from build123d import *

# Parameters (mm, degrees)
EXTRUDE_1_DEPTH   = 1018.75
FILLET_1_R        = 10
FILLET_2_R        = 8
FILLET_3_R        = 3
FILLET_4_R        = 10
FILLET_5_R        = 3
EXTRUDE_START     = 118.75
EXTRUDE_1_2_DEPTH = 118.75
EXTRUDE_2_DEPTH   = 8


with BuildPart() as part:
    # 草图1 → Extrude 1 (new body)
    with BuildSketch(Plane.XY):
        Polygon((-35, 49.6), (-35, 83.5), (35, 83.5), (35, 49.6), (15, 44.6), (15, -41.6), (67, -54.6), (67, -68.5), (-65, -68.5), (-65, -54.6), (-15, -42.1), (-15, 44.6), align=None)
    extrude(amount=EXTRUDE_1_DEPTH)

    # 圆角1
    fillet_1_edges = [part.edges().sort_by_distance(p)[0] for p in [
        (15, -41.6, 509.375),
        (-15, -42.1, 509.375),
    ]]
    fillet(fillet_1_edges, radius=FILLET_1_R)

    # 圆角2
    fillet_2_edges = [part.edges().sort_by_distance(p)[0] for p in [
        (15, 44.6, 509.375),
        (-15, 44.6, 509.375),
    ]]
    fillet(fillet_2_edges, radius=FILLET_2_R)

    # 圆角3
    fillet_3_edges = [part.edges().sort_by_distance(p)[0] for p in [
        (-35, 49.6, 509.375),
        (35, 49.6, 509.375),
    ]]
    fillet(fillet_3_edges, radius=FILLET_3_R)

    # 圆角4
    fillet_4_edges = [part.edges().sort_by_distance(p)[0] for p in [
        (-35, 83.5, 509.375),
        (35, 83.5, 509.375),
    ]]
    fillet(fillet_4_edges, radius=FILLET_4_R)

    # 圆角5
    fillet_5_edges = [part.edges().sort_by_distance(p)[0] for p in [
        (67, -54.6, 509.375),
        (-65, -54.6, 509.375),
    ]]
    fillet(fillet_5_edges, radius=FILLET_5_R)

    # 草图4 → Extrude 1 2 (add)
    with BuildSketch(Plane.XY.offset(450).offset(EXTRUDE_START)):
        with BuildLine():
            Line((142, -68.5), (142, -58.5))
            ThreePointArc((142, -58.5), (140.535533906, -54.964466094), (137, -53.5))
            Line((137, -53.5), (100.637155323, -53.5))
            ThreePointArc((100.637155323, -53.5), (97.219067588, -52.897695262), (94.212725941, -51.163335247))
            Line((94.212725941, -51.163335247), (69.787274059, -30.686664753))
            ThreePointArc((69.787274059, -30.686664753), (66.780932412, -28.952304738), (63.362844677, -28.35))
            Line((63.362844677, -28.35), (27, -28.35))
            ThreePointArc((27, -28.35), (23.464466094, -29.814466094), (22, -33.35))
            Line((22, -33.35), (22, -43.35))
            Line((22, -43.35), (64.727606875, -54.031901719))
            ThreePointArc((64.727606875, -54.031901719), (66.364616314, -55.096092591), (67, -56.942329219))
            Line((67, -56.942329219), (67, -63.5))
            ThreePointArc((67, -63.5), (68.464466094, -67.035533906), (72, -68.5))
            Line((72, -68.5), (142, -68.5))
        make_face()
    extrude_1_2 = extrude(amount=-EXTRUDE_1_2_DEPTH)

    # 草图5 → 凸台-拉伸2 (add)
    with BuildSketch(Plane(origin=(0, -53.5, 0), x_dir=(1, 0, 0), z_dir=(0, 1, 0))):
        Polygon((124.592080354, -519.375), (130.365583045, -509.375), (124.592080354, -499.375), (113.04507497, -499.375), (107.271572278, -509.375), (113.04507497, -519.375), align=None)
    extrude_2 = extrude(amount=EXTRUDE_2_DEPTH)

    # 镜向1: Extrude 1 2, 凸台-拉伸2 across plane
    add(extrude_1_2.mirror(Plane(origin=(1, 0, 0), x_dir=(0, 0, 1), z_dir=(1, 0, 0))))
    add(extrude_2.mirror(Plane(origin=(1, 0, 0), x_dir=(0, 0, 1), z_dir=(1, 0, 0))))


solid = part.part
Check sheet for the modelled part. Datum: model origin and axes. Units: mm. A direction names the side the tool comes from. Give positions to 0.01 mm unless a question says otherwise; leave off trailing zeros. Loops run counter-clockwise (first coordinate to the right, second up) from the corner with the lowest first, then second, coordinate; pieces in that order, holes last. Notation, with made-up numbers: M 6.5,-4 L 47.5,-4 A17 ccw 47.5,22 Z; hole C -22.5,24 d6. An arc over 180 degrees is marked long. Use a Markdown table: item, result. Add a question column.
Q1. Scan lines: line 1 along X through (y, z) = (28, 599); line 2 along Y through (x, z) = (-83, 535); line 3 along X through (y, z) = (-62, 339.5). Record each from-to range of solid material in increasing order. Write a range as [from, to].
Q2. Sectioned sample at B-B, the plane y = -11. Record the cut outline in (x, z).
Q3. Go/stop test with flat-tipped pins: pin 1 (10 mm diameter, centred on y = 31, z = 828.5, fed in from -X); pin 2 (6.5 mm diameter, centred on x = 121, y = -51, fed in from +Z); pin 3 (9 mm diameter, centred on y = -61, z = 285.5, fed in from -X). Record where each tip stops, or that it passes through.
Q4. Sectioned sample at A-A, the plane z = 108. Record the cut outline in (x, y).
Q5. Tool access check on faces 5 (the flat face through (-43, -28.35, 510)), 6 (the flat face through (-42.932, -49.083, 221.85)), 7 (the flat face through (45, -28.35, 510)), 8 (the flat face through (-117, -45.5, 509)), 9 (the flat face through (119, -45.5, 509)). Record the directions out of +Z, -Z, +X, -X, +Y, -Y that give a thin tool (end or side, any length) a straight path to the whole face; none if there is none.
Q6. Mould release check, pull along Y, two halves, no side actions. Record for faces 1 (the flat face through (-105, -53.5, 510)), 2 (the flat face through (43.4, -48.7, 221.8)), 3 (the flat face through (-42.932, -49.083, 790.6)), 4 (the flat face through (2, 9, 0)): pulls with the +Y half, pulls with the -Y half, needs draft (parallel to the pull), parting line crosses it, or undercut.
Verdict:
| question | item | result |
|---|---|---|
| 1 | line 1 | [-15, 15] |
| 1 | line 2 | [-68.5, -43.44] |
| 1 | line 3 | [-65, 67] |
| 2 | outline | M -15,0 L 15,0 L 15,1018.75 L -15,1018.75 Z |
| 3 | pin 1 | x = -15 |
| 3 | pin 2 | z = 568.75 |
| 3 | pin 3 | x = -65 |
| 4 | outline | M -65,-68.5 L 67,-68.5 L 67,-56.94 A3 ccw 64.73,-54.03 L 22.57,-43.49 A10 cw 15,-33.79 L 15,38.35 A8 cw 21.06,46.11 L 32.73,49.03 A3 ccw 35,51.94 L 35,73.5 A10 ccw 25,83.5 L -25,83.5 A10 ccw -35,73.5 L -35,51.94 A3 ccw -32.73,49.03 L -21.06,46.11 A8 cw -15,38.35 L -15,-34.29 A10 cw -22.57,-43.99 L -62.73,-54.03 A3 ccw -65,-56.94 Z |
| 5 | face 5 | +Z, -Z, -X |
| 5 | face 6 | -Z, -X |
| 5 | face 7 | +Z, -Z, +X |
| 5 | face 8 | +Z, -Z, -X, +Y |
| 5 | face 9 | +Z, -Z, +X, +Y |
| 6 | face 1 | pulls with the +Y half |
| 6 | face 2 | undercut |
| 6 | face 3 | undercut |
| 6 | face 4 | needs draft |
